Work out the finished part from the listing and answer in its coordinate system (mm). Round coordinates to 2 decimals unless told otherwise and drop trailing zeros. Order: outer loops, then holes, each group sorted by start corner. A loop starts at its lowest first (then second) coordinate and runs counter-clockwise, first axis right, second up. Notation, with made-up numbers: M 70.25,-3.75 L 107.25,-3.75 A8 cw 107.25,1.25 Z; hole C 31.25,-20.75 d2. An arc over 180 degrees is marked long. Return JSON: item names as keys, results as strings.
from build123d import *

# Parameters (mm, degrees)
CYLINDER001_R     = 1.5
CYLINDER001_DEPTH = 20
ARRAY_COUNT       = 8
CYLINDER_R        = 20
CYLINDER_DEPTH    = 15


with BuildPart() as array:
    # Cylinder001 → Cylinder001 (new body)
    with BuildSketch(Plane(origin=(20, 0, -2), x_dir=(1, 0, 0), z_dir=(0, 0, 1))):
        Circle(CYLINDER001_R)
    extrude(amount=CYLINDER001_DEPTH)

    # Array: Array ×8 about axis
    array_axis = Axis((0, 0, 0), (0, 0, 1))


with BuildPart() as array_1:
    add(array.part)
    for i in range(1, ARRAY_COUNT):
        add(array.part.rotate(array_axis, i * 360 / ARRAY_COUNT))


with BuildPart() as cut:
    # Cylinder → Cylinder (new body)
    with BuildSketch(Plane.XY):
        Circle(CYLINDER_R)
    extrude(amount=CYLINDER_DEPTH)

    # Cut: cut Array
    add(array_1.part, mode=Mode.SUBTRACT)


solid = cut.part
Item 1: Find section A-A (z = 11). Determine the outline of the cut face in (x, y).
Output:
{"outline": "M -19.94,-1.5 A20 ccw -15.16,-13.04 A1.5 cw -13.04,-15.16 A20 ccw -1.5,-19.94 A1.5 cw 1.5,-19.94 A20 ccw 13.04,-15.16 A1.5 cw 15.16,-13.04 A20 ccw 19.94,-1.5 A1.5 cw 19.94,1.5 A20 ccw 15.16,13.04 A1.5 cw 13.04,15.16 A20 ccw 1.5,19.94 A1.5 cw -1.5,19.94 A20 ccw -13.04,15.16 A1.5 cw -15.16,13.04 A20 ccw -19.94,1.5 A1.5 cw Z"}
Item 2: Consider line 1 along X through (y, z) = (2.5, 9.25); line 2 along Y through (x, z) = (0.5, 2.5); line 3 along Y through (x, z) = (3.5, 5.75). Determine where each line is inside the solid, lowest interval first. Write a range as [from, to].
Output:
{"line 1": "x = [-19.84, 19.84]", "line 2": "y = [-18.59, 18.59]", "line 3": "y = [-19.69, 19.69]"}
Item 3: Find section B-B (x = 0). Determine the outline of the cut face in (y, z), plus the area to 3 significant figures.
Output:
{"outline": "M -18.5,0 L 18.5,0 L 18.5,15 L -18.5,15 Z", "area": "555 mm^2"}
Item 4: Each of these flat-tipped pins is pushed along its axis until it touches: pin 1 (2 mm diameter, centred on x = 11, z = 2.5, fed in from +Y); pin 2 (2 mm diameter, centred on x = 7.5, z = 6, fed in from +Y); pin 3 (8 mm diameter, centred on x = -9.5, z = 9, fed in from -Y). Where does it stop, or does it pass through?
Output:
{"pin 1": "stops at y = 17.32", "pin 2": "stops at y = 18.91", "pin 3": "stops at y = -19.23"}
Item 5: The mould has two halves that part along Y. Classify faces 1 (the cylindrical face through (-18.44, 7.74, 7.4)), 2 (the cylindrical face through (0, -18.5, 7.4)), 3 (the cylindrical face through (13.104, -13.059, 7.395)): pulls with the +Y half, pulls with the -Y half, needs draft (parallel to the pull), parting line crosses it, or undercut.
Output:
{"face 1": "pulls with the +Y half", "face 2": "pulls with the -Y half", "face 3": "undercut"}
